from build123d import *

# Parameters (mm, degrees)
SKETCH1_W               = 10
SKETCH1_H               = 15
BOSS_EXTRUDE1_DEPTH     = 15
CUT_EXTRUDE1_DEPTH      = 18.5
CUT_EXTRUDE1_DEPTH_BACK = 18.5
SKETCH2_W               = 0.7
SKETCH2_H               = 10
SKETCH3_W               = 5
SKETCH3_H               = 2.3
BOSS_EXTRUDE2_DEPTH     = 15


with BuildPart() as part:
    # Sketch1 → Boss-Extrude1 (new body)
    with BuildSketch(Plane.XY):
        Rectangle(SKETCH1_W, SKETCH1_H)
    extrude(amount=BOSS_EXTRUDE1_DEPTH)

    # Sketch2 → Cut-Extrude1 (cut, two sides: drawn at the far end of the back side and taken through both)
    with BuildSketch(Plane.XY.offset(15).offset(-CUT_EXTRUDE1_DEPTH_BACK)):
        with Locations((0, -2.5)):
            Rectangle(SKETCH2_W, SKETCH2_H)
    extrude(amount=CUT_EXTRUDE1_DEPTH + CUT_EXTRUDE1_DEPTH_BACK, mode=Mode.SUBTRACT)

    # Sketch3 → Boss-Extrude2 (add)
    with BuildSketch(Plane.XY.offset(15)):
        with Locations((-7.5, -6.35)):
            Rectangle(SKETCH3_W, SKETCH3_H)
        with Locations((7.5, -6.35)):
            Rectangle(SKETCH3_W, SKETCH3_H)
    extrude(amount=-BOSS_EXTRUDE2_DEPTH)


solid = part.part
Could you check a few things on this model? Use its own coordinates, in mm. A direction names the side the tool comes from. Give positions to 0.01 mm unless a question says otherwise; leave off trailing zeros. Order: outer loops, then holes, each group sorted by start corner. A loop starts at its lowest first (then second) coordinate and runs counter-clockwise, first axis right, second up. Notation, with made-up numbers: (83.5, 39.5) -> (99.5, 39.5) arc R27 cw to (99.5, 77.5) -> close; hole circle Ø9 at (-37, 19.25). An arc over 180 degrees is marked (long way). Return JSON: item names as keys, results as strings.
1. Imagine slicing it at D-D on y = 4.75. List the corners of the cut face in (x, z) for me, then the cut area to 3 significant figures.
Answer list:
{"outline": "(-5, 0) -> (5, 0) -> (5, 15) -> (-5, 15) -> close", "area": "150 mm2"}
2. On a 3-axis mill with a long thin cutter (end or side, diameter ignored), from which of +Z, -Z, +X, -X, +Y, -Y can I reach the whole of each face in a straight line? I mean faces 5 (the flat face through (7, -5.2, 8)), 6 (the flat face through (-10, -6, 8)), 7 (the flat face through (-5, 1, 7)). Say none if no direction works.
Answer list:
{"face 5": "+Z, -Z, +X, +Y", "face 6": "+Z, -Z, -X, +Y, -Y", "face 7": "+Z, -Z, -X, +Y"}
3. For pin 1 Ø2.5 at (x, z) = (6.5, 7.5) entering from +Y; pin 2 Ø4 at (y, z) = (0.5, 11) entering from -X; pin 3 Ø0.6 at (x, z) = (0, 7.5) entering from -Y, each with a flat end and sliding along its axis, tell me the tip position at first contact or that it passes through.
Answer list:
{"pin 1": "stops at y = -5.2", "pin 2": "stops at x = -5", "pin 3": "stops at y = 2.5"}
4. Imagine slicing it at C-C on x = -6.5. List the corners of the cut face in (y, z) for me.
Answer list:
{"outline": "(-7.5, 0) -> (-5.2, 0) -> (-5.2, 15) -> (-7.5, 15) -> close"}
5. Thinking about a two-plate mould opening in X: for faces 1 (the flat face through (0.35, -3, 7)), 2 (the flat face through (-0.35, -3, 7)), 3 (the flat face through (5, 1, 7)), 4 (the flat face through (2, 0, 15)), which applies, pulls with the +X half, pulls with the -X half, needs draft (parallel to the pull), parting line crosses it, or undercut?
Answer list:
{"face 1": "undercut", "face 2": "undercut", "face 3": "pulls with the +X half", "face 4": "needs draft"}
6. Imagine slicing it at A-A on y = 1. List the corners of the cut face in (x, z) for me.
Answer list:
{"outline": "(-5, 0) -> (-0.35, 0) -> (-0.35, 15) -> (-5, 15) -> close; (0.35, 0) -> (5, 0) -> (5, 15) -> (0.35, 15) -> close"}
7. I need wall thicknesses on line 1 (X direction, y = -5.5, z = 12.5); line 2 (X direction, y = 0.5, z = 2); line 3 (X direction, y = 7, z = 0.75). Which ranges of each line are inside material? Lowest first, please. Write a range as from..to.
Answer list:
{"line 1": "x = -10..-0.35, 0.35..10", "line 2": "x = -5..-0.35, 0.35..5", "line 3": "x = -5..5"}
8. Imagine slicing it at B-B on z = 13. List the corners of the cut face in (x, y) for me.
Answer list:
{"outline": "(-10, -7.5) -> (-0.35, -7.5) -> (-0.35, 2.5) -> (0.35, 2.5) -> (0.35, -7.5) -> (10, -7.5) -> (10, -5.2) -> (5, -5.2) -> (5, 7.5) -> (-5, 7.5) -> (-5, -5.2) -> (-10, -5.2) -> close"}
